Read the model definition and answer for the solid it produces. Units are mm, in the model's axes. Round coordinates to 2 decimals unless told otherwise and drop trailing zeros. Write each loop counter-clockwise with the first axis right and the second up, starting at its lowest first coordinate (ties: lowest second). Pieces come first, ordered by that corner, then holes. Notation, with made-up numbers: M 87,38.25 L 126,38.25 A35 cw 126,72.25 Z; hole C -15,-39 d10. An arc over 180 degrees is marked long. Use one line per item in the form item = value. Start each with the question number.
Autodesk Inventor part; units mm, degrees
ref_plane "YZ Plane" through (0, 0, 0) normal (1, 0, 0) x (0, 1, 0)
ref_plane "XZ Plane" through (0, 0, 0) normal (0, 1, 0) x (-1, 0, 0)
ref_plane "XY Plane" through (0, 0, 0) normal (0, 0, 1) x (1, 0, 0)
sketch "スケッチ1" plane through (0, 0, 0) normal (0, 0, 1) x (1, 0, 0)
  circle A0 centre (0, 0) radius 14.05
  circle A1 centre (0, 0) radius 19.97
  circle A2 centre (0, 0) radius 14 construction
  point P0 (0, 0)
  dimension "d2" = 0.05
extrude "押し出し1" add sketch "スケッチ1" along normal blind 1
chamfer "面取り1" distance 0.4 angle 45 1 edges at (-19.97, 0, 0)
sketch "スケッチ2" plane through (0, 0, 1) normal (0, 0, 1) x (1, 0, 0)
  circle A0 centre (6.1229, -14.7821) radius 0.5915 construction
  point P0 (0, 0)
  point P1 (14.7821, -6.1229)
  point P2 (14.7821, 6.1229)
  point P3 (6.1229, 14.7821)
  point P4 (-6.1229, 14.7821)
  point P5 (-14.7821, 6.1229)
  point P6 (-14.7821, -6.1229)
  point P7 (-6.1229, -14.7821)
  dimension "d8" = 360
hole "穴1" at (6.1229, -14.7821, 1) at (14.7821, -6.1229, 1) at (14.7821, 6.1229, 1) at (6.1229, 14.7821, 1) at (-6.1229, 14.7821, 1) at (-14.7821, 6.1229, 1) at (-14.7821, -6.1229, 1) at (-6.1229, -14.7821, 1) direction (0, 0, -1) diameter 1.4 end through all countersink diameter 2.2 countersink angle 82
properties part number "UPPER_TIMING_PULLEY_COVER_INNER"
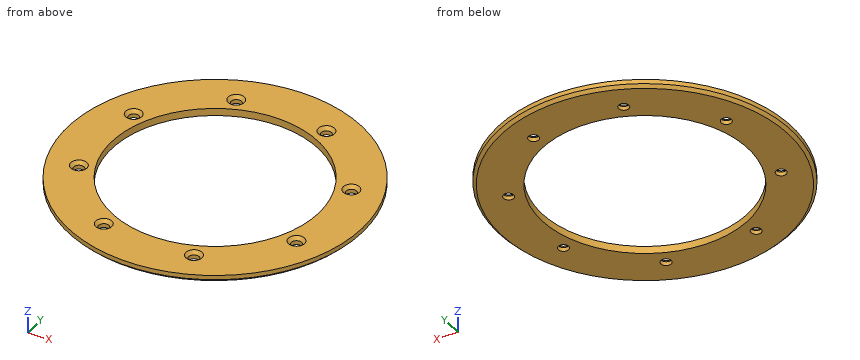
Q1. Straight lines are drawn through the part: line 1 (Y direction, x = 14.5, z = 0.6); line 2 (Y direction, x = -6.5, z = 0.45); line 3 (Y direction, x = 0, z = 0.6). For each, find the intervals that lie inside material, in ascending order. Write a range as [from, to].
Q2. Each of these flat-tipped pins is pushed along its axis until it touches: pin 1 Ø1.1 at (x, y) = (-6.12, 14.78) entering from -Z; pin 2 Ø1.6 at (x, y) = (6.12, 14.78) entering from +Z; pin 3 Ø1.8 at (x, y) = (14.78, 6.12) entering from +Z. Where does it stop, or does it pass through?
Q3. Find section A-A on x = 0. Write down the section's boundary in (y, z).
Q4. Find section C-C on z = 0.2. Count the separate pieces of the cut face and the enclosed holes in it, and give its area (3 significant figures).
Response:
q1.line_1 = [-13.73, -6.82], [-5.43, 5.43], [6.82, 13.73]
q1.line_2 = [-18.88, -15.37], [-14.19, -12.46], [12.46, 14.19], [15.37, 18.88]
q1.line_3 = [-19.97, -14.05], [14.05, 19.97]
q2.pin_1 = through
q2.pin_2 = 0.66
q2.pin_3 = 0.77
q3.outline = M -19.97,0.4 L -19.57,0 L -14.05,0 L -14.05,1 L -19.97,1 Z; M 14.05,0 L 19.57,0 L 19.97,0.4 L 19.97,1 L 14.05,1 Z
q4.separate_pieces = 1
q4.enclosed_holes = 9
q4.area = 595 mm²
